```python
from build123d import *

# Parameters (mm, degrees)
SKETCH1_R            = 12.09
SKETCH1_R_2          = 1.75
BOSS_EXTRUDE13_DEPTH = 10
SKETCH2_R            = 1.3
SKETCH2_R_2          = 2.4
CUT_EXTRUDE1_DEPTH   = 40.007683858


with BuildPart() as part:
    # Sketch1 → Boss-Extrude13 (new body)
    # profile 1 of 17: a face of its own
    with BuildSketch(Plane.XY):
        Circle(SKETCH1_R)
        Circle(SKETCH1_R_2, mode=Mode.SUBTRACT)
    # profile 2 of 17: a face of its own
    with BuildSketch(Plane.XY):
        with BuildLine():
            Line((30.75, 4), (13.976561718, 4.105641957))
            ThreePointArc((13.976561718, 4.105641957), (14.013946522, 4.095934373), (14.051260935, 4.085959636))
            Line((14.051260935, 4.085959636), (14.211728743, 3.487085624))
            ThreePointArc((14.211728743, 3.487085624), (13.144626757, 2.65424773), (11.903927815, 2.112960617))
            ThreePointArc((11.903927815, 2.112960617), (11.986568374, 1.578061664), (12.04518576, 1.04))
            ThreePointArc((12.04518576, 1.04), (13.383704325, 0.838273314), (14.63, 0.31))
            Line((14.63, 0.31), (14.63, -0.31))
            ThreePointArc((14.63, -0.31), (13.383704325, -0.838273314), (12.04518576, -1.04))
            ThreePointArc((12.04518576, -1.04), (11.986568374, -1.578061664), (11.903927815, -2.112960617))
            ThreePointArc((11.903927815, -2.112960617), (13.144626757, -2.65424773), (14.211728743, -3.487085624))
            Line((14.211728743, -3.487085624), (14.051260935, -4.085959636))
            ThreePointArc((14.051260935, -4.085959636), (14.013946522, -4.095934373), (13.976561718, -4.105641957))
            Line((13.976561718, -4.105641957), (30.75, -4))
            ThreePointArc((30.75, -4), (34.75, 0), (30.75, 4))
        make_face()
        with Locations((30.75, 0)):
            Circle(SKETCH1_R_2, mode=Mode.SUBTRACT)
    # profile 3 of 17: a face of its own
    with BuildSketch(Plane.XY):
        with BuildLine():
            ThreePointArc((-10.951436862, 5.12192646), (-10.470247132, 6.045), (-9.911436862, 6.9232593))
            ThreePointArc((-9.911436862, 6.9232593), (-11.171491285, 7.417818147), (-12.514951657, 7.583467875))
            Line((-12.514951657, 7.583467875), (-12.824951657, 7.046532125))
            ThreePointArc((-12.824951657, 7.046532125), (-12.009764599, 5.965886177), (-10.951436862, 5.12192646))
        make_face()
    # profile 4 of 17: a face of its own
    with BuildSketch(Plane.XY):
        with BuildLine():
            ThreePointArc((-9.252623584, 7.781841479), (-8.548920985, 8.548920985), (-7.781841479, 9.252623584))
            ThreePointArc((-7.781841479, 9.252623584), (-8.870959341, 10.05645683), (-10.125769107, 10.564175311))
            Line((-10.125769107, 10.564175311), (-10.564175311, 10.125769107))
            ThreePointArc((-10.564175311, 10.125769107), (-10.05645683, 8.870959341), (-9.252623584, 7.781841479))
        make_face()
    # profile 5 of 17: a face of its own
    with BuildSketch(Plane.XY):
        with BuildLine():
            ThreePointArc((-12.04518576, -1.04), (-12.09, 0), (-12.04518576, 1.04))
            ThreePointArc((-12.04518576, 1.04), (-13.383704325, 0.838273314), (-14.63, 0.31))
            Line((-14.63, 0.31), (-14.63, -0.31))
            ThreePointArc((-14.63, -0.31), (-13.383704325, -0.838273314), (-12.04518576, -1.04))
        make_face()
    # profile 6 of 17: a face of its own
    with BuildSketch(Plane.XY):
        with BuildLine():
            ThreePointArc((-11.903927815, 2.112960617), (-11.67804324, 3.129122255), (-11.365584201, 4.122086336))
            ThreePointArc((-11.365584201, 4.122086336), (-12.71070456, 4.273667417), (-14.051260935, 4.085959636))
            Line((-14.051260935, 4.085959636), (-14.211728743, 3.487085624))
            ThreePointArc((-14.211728743, 3.487085624), (-13.144626757, 2.65424773), (-11.903927815, 2.112960617))
        make_face()
    # profile 7 of 17: a face of its own
    with BuildSketch(Plane.XY):
        with BuildLine():
            ThreePointArc((-6.9232593, 9.911436862), (-6.045, 10.470247132), (-5.12192646, 10.951436862))
            ThreePointArc((-5.12192646, 10.951436862), (-5.965886177, 12.009764599), (-7.046532125, 12.824951657))
            Line((-7.046532125, 12.824951657), (-7.583467875, 12.514951657))
            ThreePointArc((-7.583467875, 12.514951657), (-7.417818147, 11.171491285), (-6.9232593, 9.911436862))
        make_face()
    # profile 8 of 17: a face of its own
    with BuildSketch(Plane.XY):
        with BuildLine():
            ThreePointArc((12.514951657, 7.583467875), (11.171491285, 7.417818147), (9.911436862, 6.9232593))
            ThreePointArc((9.911436862, 6.9232593), (10.470247132, 6.045), (10.951436862, 5.12192646))
            ThreePointArc((10.951436862, 5.12192646), (12.009764599, 5.965886177), (12.824951657, 7.046532125))
            Line((12.824951657, 7.046532125), (12.514951657, 7.583467875))
        make_face()
    # profile 9 of 17: a face of its own
    with BuildSketch(Plane.XY):
        with BuildLine():
            ThreePointArc((10.125769107, 10.564175311), (8.870959341, 10.05645683), (7.781841479, 9.252623584))
            ThreePointArc((7.781841479, 9.252623584), (8.548920985, 8.548920985), (9.252623584, 7.781841479))
            ThreePointArc((9.252623584, 7.781841479), (10.05645683, 8.870959341), (10.564175311, 10.125769107))
            Line((10.564175311, 10.125769107), (10.125769107, 10.564175311))
        make_face()
    # profile 10 of 17: a face of its own
    with BuildSketch(Plane.XY):
        with BuildLine():
            ThreePointArc((7.046532125, 12.824951657), (5.965886177, 12.009764599), (5.12192646, 10.951436862))
            ThreePointArc((5.12192646, 10.951436862), (6.045, 10.470247132), (6.9232593, 9.911436862))
            ThreePointArc((6.9232593, 9.911436862), (7.417818147, 11.171491285), (7.583467875, 12.514951657))
            Line((7.583467875, 12.514951657), (7.046532125, 12.824951657))
        make_face()
    # profile 11 of 17: a face of its own
    with BuildSketch(Plane.XY):
        with BuildLine():
            ThreePointArc((3.487085624, 14.211728743), (2.65424773, 13.144626757), (2.112960617, 11.903927815))
            ThreePointArc((2.112960617, 11.903927815), (3.129122255, 11.67804324), (4.122086336, 11.365584201))
            ThreePointArc((4.122086336, 11.365584201), (4.273667417, 12.71070456), (4.085959636, 14.051260935))
            Line((4.085959636, 14.051260935), (3.487085624, 14.211728743))
        make_face()
    # profile 12 of 17: a face of its own
    with BuildSketch(Plane.XY):
        with BuildLine():
            ThreePointArc((1.04, 12.04518576), (0.838273314, 13.383704325), (0.31, 14.63))
            Line((0.31, 14.63), (-0.31, 14.63))
            ThreePointArc((-0.31, 14.63), (-0.838273314, 13.383704325), (-1.04, 12.04518576))
            ThreePointArc((-1.04, 12.04518576), (0, 12.09), (1.04, 12.04518576))
        make_face()
    # profile 13 of 17: a face of its own
    with BuildSketch(Plane.XY):
        with BuildLine():
            ThreePointArc((-4.122086336, 11.365584201), (-3.129122255, 11.67804324), (-2.112960617, 11.903927815))
            ThreePointArc((-2.112960617, 11.903927815), (-2.65424773, 13.144626757), (-3.487085624, 14.211728743))
            Line((-3.487085624, 14.211728743), (-4.085959636, 14.051260935))
            ThreePointArc((-4.085959636, 14.051260935), (-4.273667417, 12.71070456), (-4.122086336, 11.365584201))
        make_face()
    # profile 14 of 17: a face of its own
    with BuildSketch(Plane.XY):
        with BuildLine():
            Line((13.976561718, 4.105641957), (11.365584201, 4.122086336))
            ThreePointArc((11.365584201, 4.122086336), (11.67804324, 3.129122255), (11.903927815, 2.112960617))
            ThreePointArc((11.903927815, 2.112960617), (13.144626757, 2.65424773), (14.211728743, 3.487085624))
            Line((14.211728743, 3.487085624), (14.051260935, 4.085959636))
            ThreePointArc((14.051260935, 4.085959636), (14.013946522, 4.095934373), (13.976561718, 4.105641957))
        make_face()
    # profile 15 of 17: a face of its own
    with BuildSketch(Plane.XY):
        with BuildLine():
            ThreePointArc((14.63, 0.31), (13.383704325, 0.838273314), (12.04518576, 1.04))
            ThreePointArc((12.04518576, 1.04), (12.078791244, 0.520482544), (12.09, 0))
            ThreePointArc((12.09, 0), (12.078791244, -0.520482544), (12.04518576, -1.04))
            ThreePointArc((12.04518576, -1.04), (13.383704325, -0.838273314), (14.63, -0.31))
            Line((14.63, -0.31), (14.63, 0.31))
        make_face()
    # profile 16 of 17: a face of its own
    with BuildSketch(Plane.XY):
        with BuildLine():
            Line((11.365584201, -4.122086336), (13.976561718, -4.105641957))
            ThreePointArc((13.976561718, -4.105641957), (14.013946522, -4.095934373), (14.051260935, -4.085959636))
            Line((14.051260935, -4.085959636), (14.211728743, -3.487085624))
            ThreePointArc((14.211728743, -3.487085624), (13.144626757, -2.65424773), (11.903927815, -2.112960617))
            ThreePointArc((11.903927815, -2.112960617), (11.67804324, -3.129122255), (11.365584201, -4.122086336))
        make_face()
    # profile 17 of 17: a face of its own
    with BuildSketch(Plane.XY):
        with BuildLine():
            ThreePointArc((-11.365584201, -4.122086336), (-11.67804324, -3.129122255), (-11.903927815, -2.112960617))
            ThreePointArc((-11.903927815, -2.112960617), (-13.144626757, -2.65424773), (-14.211728743, -3.487085624))
            Line((-14.211728743, -3.487085624), (-14.051260935, -4.085959636))
            ThreePointArc((-14.051260935, -4.085959636), (-12.71070456, -4.273667417), (-11.365584201, -4.122086336))
        make_face()
    extrude(amount=BOSS_EXTRUDE13_DEPTH)

    # Sketch2 → Cut-Extrude1 (cut, through all)
    with BuildSketch(Plane.XY.offset(10)):
        with Locations((-4.5, 0)):
            Circle(SKETCH2_R)
        with Locations((4.5, 0)):
            Circle(SKETCH2_R)
        Circle(SKETCH2_R_2)
    extrude(amount=-CUT_EXTRUDE1_DEPTH, mode=Mode.SUBTRACT)


solid = part.part
```
Read the model definition and answer for the solid it produces. Units are mm, in the model's axes. A direction names the side the tool comes from. Round coordinates to 2 decimals unless told otherwise and drop trailing zeros. Loops run counter-clockwise (first coordinate to the right, second up) from the corner with the lowest first, then second, coordinate; pieces in that order, holes last. Notation, with made-up numbers: (79, 50) -> (134, 50) arc R32 cw to (134, 78) -> close; hole circle Ø4 at (16.25, -31.5). An arc over 180 degrees is marked (long way). One line per item, written item: value.
1) Consider L1, parallel to X at y = 12.5, z = 3.5; L2, parallel to X at y = -1.5, z = 2.75; L3, parallel to Y at x = 30.75, z = 5. Determine where each line is inside the solid, lowest interval first. Write a range as [from, to].
Answer list:
L1: x = [-7.58, -6.55], [-4.27, -2.33], [-1.01, 1.01], [2.33, 4.27], [6.55, 7.58]
L2: x = [-12, -1.87], [1.87, 29.85], [31.65, 34.46]
L3: y = [-4, -1.75], [1.75, 4]
2) A cutting plane is placed at B-B (z = 8.75). Give the number of separate pieces and of enclosed holes in the cut face, and give its area (3 significant figures).
Answer list:
separate pieces: 1
enclosed holes: 4
area: 648 mm²
3) Flat-ended cylindrical pins translate along their axes: P1, Ø6, axis at x = 4.5, z = 4, coming from the +Y side; P2, Ø1, axis at x = 8, z = 1, coming from the +Y side; P3, Ø5, axis at y = 5, z = 4, coming from the +X side. Find the tip coordinate at first contact, or state that the pin passes through.
Answer list:
P1: stops at y = 14.21
P2: stops at y = 12.56
P3: stops at x = 33.87
4) A cutting plane is placed at C-C (x = 22). Determine the outline of the cut face in (y, z).
Answer list:
outline: (-4.06, 0) -> (4.06, 0) -> (4.06, 10) -> (-4.06, 10) -> close
5) For faces 5 (the face through (-8.854, 10.047, 4.93)), 6 (the face through (11.996, 5.952, 4.93)), 7 (the face through (-11.988, -1.571, 4.93)), 8 (the face through (-7.35, 9.6, 4.93)), determine the directions among +Z, -Z, +X, -X, +Y, -Y from which every point of the face is accessible in a straight line to the end or side of a thin tool.
Answer list:
face 5: +Z, -Z, +Y
face 6: +Z, -Z, +X
face 7: +Z, -Z, -X
face 8: +Z, -Z
6) A cutting plane is placed at A-A (x = 30). Determine the outline of the cut face in (y, z).
Answer list:
outline: (-4, 0) -> (-1.58, 0) -> (-1.58, 10) -> (-4, 10) -> close; (1.58, 0) -> (4, 0) -> (4, 10) -> (1.58, 10) -> close
7) The mould has two halves that part along Y. Classify faces 1 (the face through (7.366, 9.587, 4.93)), 2 (the face through (-0.833, 13.402, 4.93)), 3 (the face through (29, 0, 5)), 4 (the face through (-0.21, -12.09, 4.93)): pulls with the +Y half, pulls with the -Y half, needs draft (parallel to the pull), parting line crosses it, or undercut.
Answer list:
face 1: undercut
face 2: pulls with the +Y half
face 3: undercut
face 4: pulls with the -Y half
